Answer from the drawing. Dimensions are ordinates in mm from the lowest x, y and z of the part. A direction names the side the tool comes from. Coordinates: 2 decimals unless noted, no trailing zeros. Order: outer loops, then holes, each group sorted by start corner. A loop starts at its lowest first (then second) coordinate and runs counter-clockwise, first axis right, second up. Notation, with made-up numbers: (36.5, 28) - (55.5, 28) arc R29 cw to (55.5, 53) - close; hole circle Ø5 at (56.5, 19). An arc over 180 degrees is marked (long way). Answer as a JSON object with one key per item and string values. Group by question number.
1) The mould has two halves that part along X. Classify the marked faces 1, 2 and 3: released by +X, released by -X, zero draft, split by the parting line, or undercut.
2) Section C-C (x = 13) is taken. Give the vertices of the cut face in (y, z), plus the area to 3 significant figures.
3) Section B-B (y = 12.25) is taken. Give the vertices of the cut face in (x, z), plus the area to 3 significant figures.
4) Find the intervals of material crossed by line 1 along Y through (x, z) = (48, 3); line 2 along X through (y, z) = (18.25, 15.75); line 3 along X through (y, z) = (11.75, 8.75), in increasing order.
5) Each of these flat-tipped pins is pushed along its axis until it touches: P1, Ø2.5, axis at y = 13.5, z = 14, coming from the -X side; P2, Ø3, axis at x = 24, y = 16, coming from the +Z side. Where does it stop, or does it pass through?
6) Section A-A (z = 15.5) is taken. Give the vertices of the cut face in (x, y), plus the area to 3 significant figures.
7) A tool of negligible diameter and unlimited length cuts with its end or side. For the marked faces 4 and 5, from which of +Z, -Z, +X, -X, +Y, -Y can it reach the whole face along a straight path? Write none if from no direction.
8) Section D-D (y = 6.25) is taken. Give the vertices of the cut face in (x, z), plus the area to 4 significant figures.
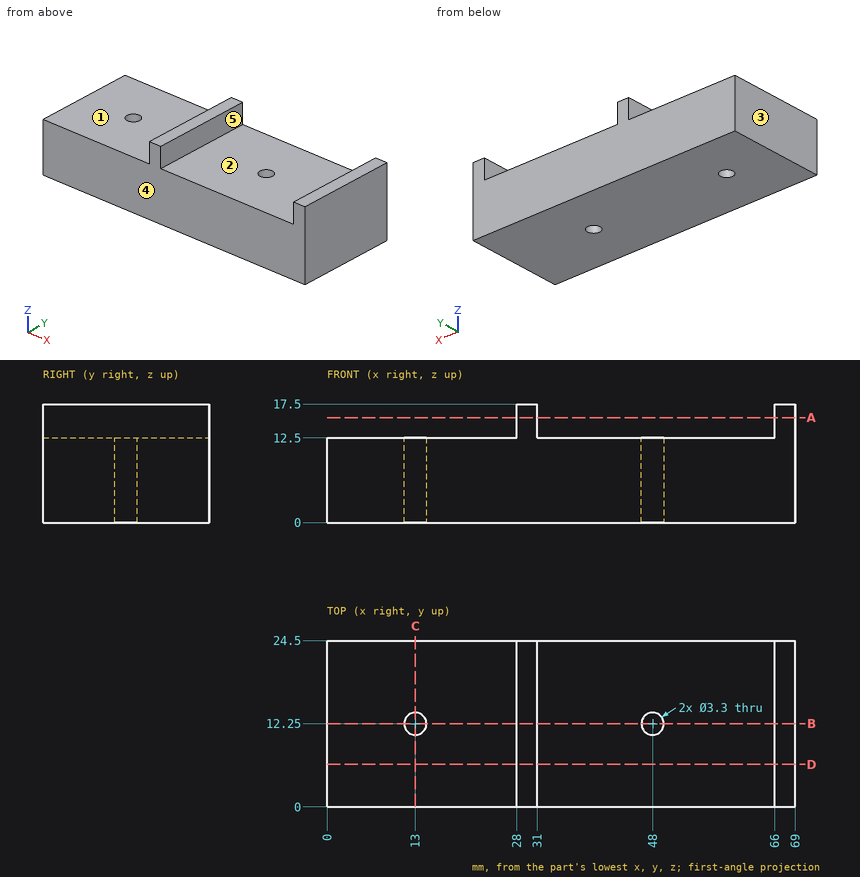
Report:
{
 "1": {"face 1": "zero draft", "face 2": "undercut", "face 3": "released by -X"},
 "2": {"outline": "(0, 0) - (10.6, 0) - (10.6, 12.5) - (0, 12.5) - close; (13.9, 0) - (24.5, 0) - (24.5, 12.5) - (13.9, 12.5) - close", "area": "265 mm²"},
 "3": {"outline": "(0, 0) - (11.35, 0) - (11.35, 12.5) - (0, 12.5) - close; (14.65, 0) - (46.35, 0) - (46.35, 12.5) - (31, 12.5) - (31, 17.5) - (28, 17.5) - (28, 12.5) - (14.65, 12.5) - close; (49.65, 0) - (69, 0) - (69, 17.5) - (66, 17.5) - (66, 12.5) - (49.65, 12.5) - close", "area": "810 mm²"},
 "4": {"line 1": "y = 0 to 10.6, 13.9 to 24.5", "line 2": "x = 28 to 31, 66 to 69", "line 3": "x = 0 to 11.43, 14.57 to 46.43, 49.57 to 69"},
 "5": {"P1": "stops at x = 28", "P2": "stops at z = 12.5"},
 "6": {"outline": "(28, 0) - (31, 0) - (31, 24.5) - (28, 24.5) - close; (66, 0) - (69, 0) - (69, 24.5) - (66, 24.5) - close", "area": "147 mm²"},
 "7": {"face 4": "+Z, -Z, +X, -X, -Y", "face 5": "+Z, +Y, -Y"},
 "8": {"outline": "(0, 0) - (69, 0) - (69, 17.5) - (66, 17.5) - (66, 12.5) - (31, 12.5) - (31, 17.5) - (28, 17.5) - (28, 12.5) - (0, 12.5) - close", "area": "892.5 mm²"}
}
